For this review, use the dimensioned drawing (mm, ordinates from the lowest corner) and the shaded views. Coordinates: 2 decimals unless noted, no trailing zeros. Loops run counter-clockwise (first coordinate to the right, second up) from the corner with the lowest first, then second, coordinate; pieces in that order, holes last. Notation, with made-up numbers: M 80.25,86.25 L 120.25,86.25 A18 cw 120.25,117.25 Z; hole C -2.75,-34.75 d11. An arc over 180 degrees is marked long. One line per item, written item: value.
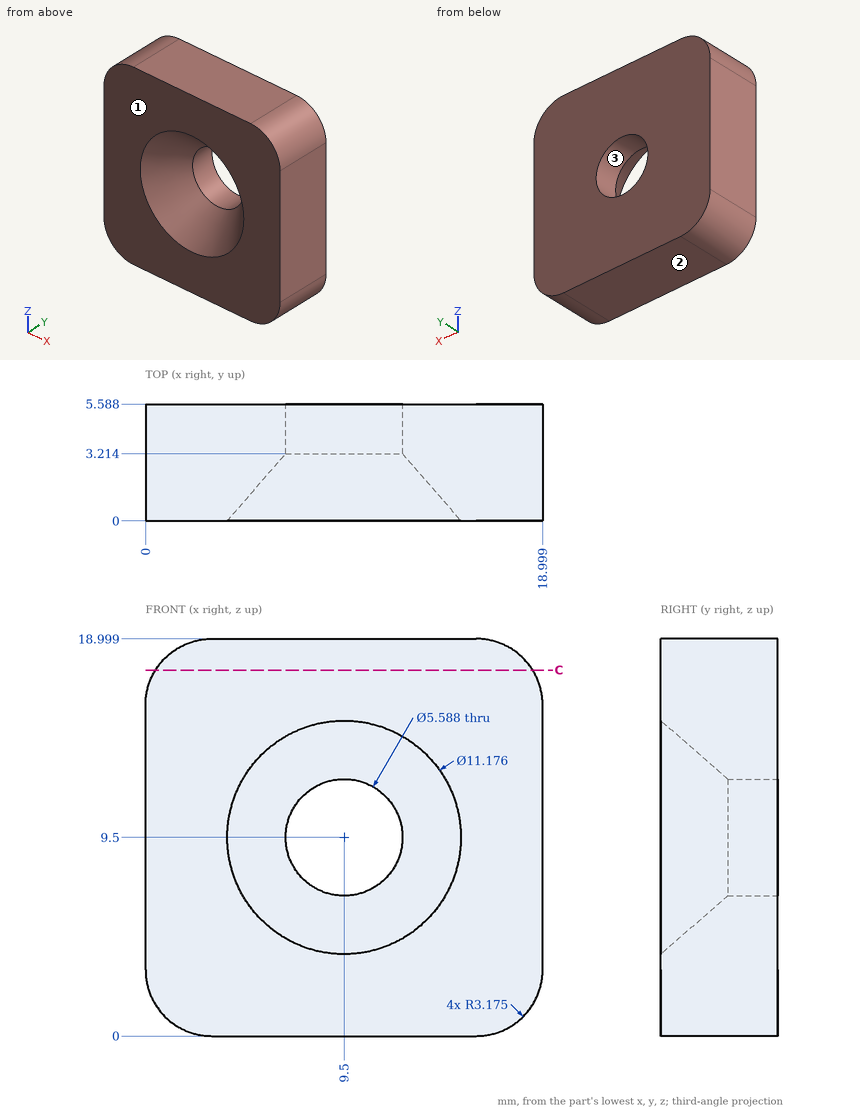
(1) To check wall thickness, follow line 1 along X through (y, z) = (1.7, 3) (1 decimal); line 2 along Z through (x, y) = (13.75, 0.8) (1 decimal); line 3 along Z through (x, y) = (7.75, 2.3) (1 decimal). State the ranges of each line that lie inside material, in increasing order. Write a range as [from, to].
Reply:
line 1: x = [0, 19]
line 2: z = [0, 7.1], [11.9, 19]
line 3: z = [0, 6.4], [12.6, 19]
(2) We need section C-C on z = 17.5. State the section outline as (x, y) points.
Reply:
outline: M 0.48,0 L 18.52,0 L 18.52,5.59 L 0.48,5.59 Z
(3) Insertion check: pin 1 (1.5 mm diameter, centred on x = 11, z = 10, fed in from -Y); pin 2 (5 mm diameter, centred on x = 10, z = 9, fed in from -Y). Each pin has a flat end and moves straight along its axis. Give the tip position at first contact, or say it passes through.
Reply:
pin 1: passes through
pin 2: stops at y = 2.74
(4) Mouldability with a two-part tool opening along Z and no side actions: class the marked faces 1, 2 and 3 as released by +Z, released by -Z, zero draft, split by the parting line, or undercut.
Reply:
face 1: zero draft
face 2: released by -Z
face 3: undercut
